The model under review builds one solid part; all positions refer to its coordinate system, in mm. A direction names the side the tool comes from. Coordinates: 2 decimals unless noted, no trailing zeros. Order: outer loops, then holes, each group sorted by start corner. A loop starts at its lowest first (then second) coordinate and runs counter-clockwise, first axis right, second up. Notation, with made-up numbers: (65, 22.25) -> (96, 22.25) arc R27 cw to (96, 60.25) -> close; hole circle Ø7 at (63.25, 16.5). An arc over 180 degrees is marked (long way). Answer as CSV lines item,"result". Start each with the question number.
from build123d import *

# Parameters (mm, degrees)
SKETCH1_W               = 60
SKETCH1_H               = 15
BOSS_EXTRUDE1_DEPTH     = 10
BOSS_EXTRUDE2_DEPTH     = 60
SKETCH3_R               = 1.25
CUT_EXTRUDE1_DEPTH      = 1
CUT_EXTRUDE1_DEPTH_BACK = 16


with BuildPart() as part:
    # Sketch1 → Boss-Extrude1 (new body)
    with BuildSketch(Plane.XY):
        Rectangle(SKETCH1_W, SKETCH1_H)
    extrude(amount=BOSS_EXTRUDE1_DEPTH)

    # Sketch2 → Boss-Extrude2 (add)
    with BuildSketch(Plane(origin=(30, 0, 0), x_dir=(0, 0, -1), z_dir=(1, 0, 0))):
        Polygon((0, 4), (4.124819933, 6), (4.124819933, -6), (0, -4), align=None)
    extrude(amount=-BOSS_EXTRUDE2_DEPTH)

    # Sketch3 → Cut-Extrude1 (cut, two sides)
    with BuildSketch(Plane(origin=(0, 7.5, 0), x_dir=(1, 0, 0), z_dir=(0, 1, 0))) as cut_extrude1_sk:
        with Locations((-22, -5)):
            Circle(SKETCH3_R)
        with Locations((22, -5)):
            Circle(SKETCH3_R)
    extrude(amount=CUT_EXTRUDE1_DEPTH, mode=Mode.SUBTRACT)
    extrude(cut_extrude1_sk.sketch, amount=-CUT_EXTRUDE1_DEPTH_BACK, mode=Mode.SUBTRACT)


solid = part.part
1) Consider section A-A (x = -22). Give the boundary of the cut face in (y, z), plus the area to 3 significant figures.
2) Insertion check: pin 1 Ø1.5 at (x, z) = (22, 5) entering from +Y; pin 2 Ø2 at (y, z) = (-6, -2.5) entering from -X. Each pin has a flat end and moves straight along its axis. Give the tip position at first contact, or say it passes through.
3) Mouldability with a two-part tool opening along X and no side actions: class faces 4 (the face through (-30, 0, 3)), 5 (the face through (-20.845, 0.105, 5.479)), 6 (the face through (0, 7.5, 5)) as released by +X, released by -X, zero draft, split by the parting line, or undercut.
4) Consider section B-B (x = -6.5). Give the boundary of the cut face in (y, z), plus the area to 3 significant figures.
5) Tool access review of faces 1 (the face through (0, -6, 0)), 2 (the face through (0, 0, -4.125)), 3 (the face through (0.42, 4.986, -2.034)): name each direction out of +Z, -Z, +X, -X, +Y, -Y from which nothing blocks a thin tool from reaching the whole face with its end or side.
6) Wall thickness on L1, parallel to X at y = -1.25, z = 5; L2, parallel to Z at x = -22, y = -3.5; L3, parallel to Z at x = 13, y = 7: over which ranges is each line inside the solid? List them lowest first. Write a range as [from, to].
Result:
1,outline,"(-7.5, 0) -> (-4, 0) -> (-6, -4.12) -> (6, -4.12) -> (4, 0) -> (7.5, 0) -> (7.5, 3.75) -> (-7.5, 3.75) -> close; (-7.5, 6.25) -> (7.5, 6.25) -> (7.5, 10) -> (-7.5, 10) -> close"
1,area,"154 mm2"
2,pin 1,"through"
2,pin 2,"x = -30"
3,face 4,"released by -X"
3,face 5,"undercut"
3,face 6,"zero draft"
4,outline,"(-7.5, 0) -> (-4, 0) -> (-6, -4.12) -> (6, -4.12) -> (4, 0) -> (7.5, 0) -> (7.5, 10) -> (-7.5, 10) -> close"
4,area,"191 mm2"
5,face 1,"+X, -X, -Y"
5,face 2,"-Z, +X, -X, +Y, -Y"
5,face 3,"+X, -X, +Y"
6,L1,"[-30, -23.25], [-20.75, 20.75], [23.25, 30]"
6,L2,"[-4.12, 3.75], [6.25, 10]"
6,L3,"[0, 10]"
